from build123d import *

# Parameters (mm, degrees)
BOSS_EXTRUDE1_DEPTH     = 32.5
SKETCH4_R               = 1.05
BOSS_EXTRUDE2_DEPTH     = 2.5
SKETCH5_R               = 1.05
BOSS_EXTRUDE3_DEPTH     = 3
CUT_EXTRUDE1_DEPTH      = 31.122
SKETCH13_W              = 30.122
SKETCH13_H              = 38
BOSS_EXTRUDE7_DEPTH     = 2.5
BOSS_EXTRUDE4_DEPTH     = 5
BOSS_EXTRUDE6_DEPTH     = 5
CUT_EXTRUDE2_DEPTH      = 6
SKETCH14_W              = 15
SKETCH14_H              = 5
CUT_EXTRUDE3_DEPTH      = 11
SKETCH15_W              = 30.122
SKETCH15_H              = 34.5
SKETCH15_R              = 2.495
BOSS_EXTRUDE8_DEPTH     = 3
SKETCH17_R              = 13.75
CUT_EXTRUDE4_DEPTH      = 53
SKETCH19_W              = 15
SKETCH19_H              = 3
CUT_EXTRUDE6_DEPTH      = 30.5
CUT_EXTRUDE6_DEPTH_BACK = 11
SKETCH21_R              = 2.25
CUT_EXTRUDE8_DEPTH      = 1.5
SKETCH20_R              = 10
CUT_EXTRUDE7_DEPTH      = 6
CHAMFER1_SIZE           = 2
CHAMFER1_SIZE2          = 1.154700538
CHAMFER1_PART_2_SIZE    = 2
CHAMFER1_PART_2_SIZE2   = 1.154700538
CHAMFER1_PART_3_SIZE    = 2
CHAMFER1_PART_3_SIZE2   = 1.154700538
CHAMFER1_PART_4_SIZE    = 2
CHAMFER1_PART_4_SIZE2   = 1.154700538
CHAMFER1_PART_5_SIZE    = 2
CHAMFER1_PART_5_SIZE2   = 1.154700538
CHAMFER1_PART_6_SIZE    = 2
CHAMFER1_PART_6_SIZE2   = 1.154700538
CHAMFER1_PART_7_SIZE    = 2
CHAMFER1_PART_7_SIZE2   = 1.154700538
CHAMFER1_PART_8_SIZE    = 2
CHAMFER1_PART_8_SIZE2   = 1.154700538
CHAMFER1_PART_9_SIZE    = 2
CHAMFER1_PART_9_SIZE2   = 1.154700538
CHAMFER1_PART_10_SIZE   = 2
CHAMFER1_PART_10_SIZE2  = 1.154700538
CHAMFER1_PART_11_SIZE   = 2
CHAMFER1_PART_11_SIZE2  = 1.154700538
CHAMFER1_PART_12_SIZE   = 2
CHAMFER1_PART_12_SIZE2  = 1.154700538
CHAMFER1_PART_13_SIZE   = 2
CHAMFER1_PART_13_SIZE2  = 1.154700538
CHAMFER1_PART_14_SIZE   = 2
CHAMFER1_PART_14_SIZE2  = 1.154700538
CHAMFER1_PART_15_SIZE   = 2
CHAMFER1_PART_15_SIZE2  = 1.154700538
CHAMFER1_PART_16_SIZE   = 2
CHAMFER1_PART_16_SIZE2  = 1.154700538
CHAMFER1_PART_17_SIZE   = 2
CHAMFER1_PART_17_SIZE2  = 1.154700538
CHAMFER1_PART_18_SIZE   = 2
CHAMFER1_PART_18_SIZE2  = 1.154700538


with BuildPart() as part:
    # Sketch2 → Boss-Extrude1 (new body)
    with BuildSketch(Plane(origin=(0, 0, 0), x_dir=(1, 0, 0), z_dir=(0, 1, 0))):
        Polygon((15.061, 0), (15.061, 32), (12.561, 32), (12.561, 2.5), (-12.561, 2.5), (-12.561, 32), (-15.061, 32), (-15.061, 0), align=None)
    extrude(amount=BOSS_EXTRUDE1_DEPTH)

    # Sketch4 → Boss-Extrude2 (add)
    with BuildSketch(Plane.XZ):
        Polygon((-7.561, -6), (-7.561, 0), (-15.061, 0), (-15.061, -32), (-12.561, -32), (-12.561, -10), align=None)
        with Locations((-10.2499, -4.95)):
            Circle(SKETCH4_R, mode=Mode.SUBTRACT)
        Polygon((12.561, -10), (7.561, -6), (7.561, 0), (15.061, 0), (15.061, -32), (12.561, -32), align=None)
        with Locations((10.2499, -4.95)):
            Circle(SKETCH4_R, mode=Mode.SUBTRACT)
    extrude(amount=BOSS_EXTRUDE2_DEPTH)

    # Sketch5 → Boss-Extrude3 (add)
    with BuildSketch(Plane(origin=(0, 32.5, 0), x_dir=(1, 0, 0), z_dir=(0, 1, 0))):
        Polygon((-15.061, 32), (-10.2499, 32), (-6.25, 26), (6.25, 26), (10.2499, 32), (15.061, 32), (15.061, 0), (-15.061, 0), align=None)
        with Locations((-10.2499, 8.7)):
            Circle(SKETCH5_R, mode=Mode.SUBTRACT)
        with Locations((10.2499, 8.7)):
            Circle(SKETCH5_R, mode=Mode.SUBTRACT)
    extrude(amount=BOSS_EXTRUDE3_DEPTH)

    # Sketch6 → Cut-Extrude1 (cut, through all)
    with BuildSketch(Plane.ZY.offset(15.061)):
        Polygon((-12.5, 35.5), (-32, 2.5), (-32, 35.5), align=None)
    extrude(amount=-CUT_EXTRUDE1_DEPTH, mode=Mode.SUBTRACT)

    # Sketch13 → Boss-Extrude7 (add)
    with BuildSketch(Plane.XY):
        with Locations((0, 16.5)):
            Rectangle(SKETCH13_W, SKETCH13_H)
    extrude(amount=BOSS_EXTRUDE7_DEPTH)

    # Sketch8 → Boss-Extrude4 (add)
    with BuildSketch(Plane.XY.offset(2.5)):
        Polygon((0, -43.5), (-43.59255168, 16.5), (43.59255168, 16.5), align=None)
    extrude(amount=BOSS_EXTRUDE4_DEPTH)

    # Sketch9 → Boss-Extrude6 (add)
    with BuildSketch(Plane.XY.offset(2.5)):
        Polygon((43.59255168, 16.5), (65.38882752, 46.5), (-65.38882752, 46.5), (-43.59255168, 16.5), align=None)
    extrude(amount=BOSS_EXTRUDE6_DEPTH)

    # Sketch10 → Cut-Extrude2 (cut, through all)
    with BuildSketch(Plane(origin=(0, 0, 2.5), x_dir=(-1, 0, 0), z_dir=(0, 0, -1))):
        Polygon((-25.38882752, 46.5), (-65.38882752, 46.5), (-41.877417429, 14.139320225), align=None)
        Polygon((65.38882752, 46.5), (41.877417429, 14.139320225), (25.38882752, 46.5), align=None)
    extrude(amount=-CUT_EXTRUDE2_DEPTH, mode=Mode.SUBTRACT)

    # Sketch14 → Cut-Extrude3 (cut, through all)
    with BuildSketch(Plane(origin=(0, 0, -2.5), x_dir=(-1, 0, 0), z_dir=(0, 0, -1))):
        Polygon((-7.561, -2.5), (7.561, -2.5), (7.561, 0), (12.561, 0), (12.561, 7.783674653), (-12.561, 7.783674653), (-12.561, 0), (-7.561, 0), align=None)
        with Locations((0, 38)):
            Rectangle(SKETCH14_W, SKETCH14_H)
    extrude(amount=-CUT_EXTRUDE3_DEPTH, mode=Mode.SUBTRACT)

    # Sketch15 → Boss-Extrude8 (add)
    with BuildSketch(Plane.XZ.offset(2.5)):
        with Locations((0, -14.75)):
            Rectangle(SKETCH15_W, SKETCH15_H)
        with Locations((-10.2499, -4.95)):
            Circle(SKETCH15_R, mode=Mode.SUBTRACT)
        with Locations((10.340989886, -4.95)):
            Circle(SKETCH15_R, mode=Mode.SUBTRACT)
    extrude(amount=BOSS_EXTRUDE8_DEPTH)

    # Sketch17 → Cut-Extrude4 (cut, through all)
    with BuildSketch(Plane.XZ.offset(5.5)):
        with Locations((0, -37.5)):
            Circle(SKETCH17_R)
    extrude(amount=-CUT_EXTRUDE4_DEPTH, mode=Mode.SUBTRACT)

    # Sketch19 → Cut-Extrude6 (cut, two sides)
    with BuildSketch(Plane(origin=(0, 0, -2.5), x_dir=(-1, 0, 0), z_dir=(0, 0, -1))) as cut_extrude6_sk:
        with Locations((0, 34)):
            Rectangle(SKETCH19_W, SKETCH19_H)
    extrude(amount=CUT_EXTRUDE6_DEPTH, mode=Mode.SUBTRACT)
    extrude(cut_extrude6_sk.sketch, amount=-CUT_EXTRUDE6_DEPTH_BACK, mode=Mode.SUBTRACT)

    # Sketch21 → Cut-Extrude8 (cut)
    with BuildSketch(Plane(origin=(0, 35.5, 0), x_dir=(1, 0, 0), z_dir=(0, 1, 0))):
        with Locations((-10.2499, 8.7)):
            Circle(SKETCH21_R)
        with Locations((10.2499, 8.7)):
            Circle(SKETCH21_R)
    extrude(amount=-CUT_EXTRUDE8_DEPTH, mode=Mode.SUBTRACT)

    # Sketch20 → Cut-Extrude7 (cut, through all)
    with BuildSketch(Plane(origin=(0, 0, 2.5), x_dir=(-1, 0, 0), z_dir=(0, 0, -1))):
        with Locations((0, -43.5)):
            Circle(SKETCH20_R)
    extrude(amount=-CUT_EXTRUDE7_DEPTH, mode=Mode.SUBTRACT)

    # Chamfer1
    chamfer1_edges = [part.edges().sort_by_distance(p)[0] for p in [
        (-23.877634976, -10.635254916, 7.5),
    ]]
    chamfer1_side = [part.faces().sort_by_distance(p)[0] for p in [
        (-23.877634976, -10.635254916, 5),
    ]]
    chamfer(chamfer1_edges, length=CHAMFER1_SIZE, length2=CHAMFER1_SIZE2, reference=chamfer1_side[0])

    # Chamfer1 part 2
    chamfer1_part_2_edges = [part.edges().sort_by_distance(p)[0] for p in [
        (-33.633122475, 30.319660113, 7.5),
    ]]
    chamfer1_part_2_side = [part.faces().sort_by_distance(p)[0] for p in [
        (-33.633122475, 30.319660113, 5),
    ]]
    chamfer(chamfer1_part_2_edges, length=CHAMFER1_PART_2_SIZE, length2=CHAMFER1_PART_2_SIZE2, reference=chamfer1_part_2_side[0])

    # Chamfer1 part 3
    chamfer1_part_3_edges = [part.edges().sort_by_distance(p)[0] for p in [
        (0, 46.5, 7.5),
    ]]
    chamfer1_part_3_side = [part.faces().sort_by_distance(p)[0] for p in [
        (0, 46.5, 5),
    ]]
    chamfer(chamfer1_part_3_edges, length=CHAMFER1_PART_3_SIZE, length2=CHAMFER1_PART_3_SIZE2, reference=chamfer1_part_3_side[0])

    # Chamfer1 part 4
    chamfer1_part_4_edges = [part.edges().sort_by_distance(p)[0] for p in [
        (33.633122475, 30.319660113, 7.5),
    ]]
    chamfer1_part_4_side = [part.faces().sort_by_distance(p)[0] for p in [
        (33.633122475, 30.319660113, 5),
    ]]
    chamfer(chamfer1_part_4_edges, length=CHAMFER1_PART_4_SIZE, length2=CHAMFER1_PART_4_SIZE2, reference=chamfer1_part_4_side[0])

    # Chamfer1 part 5
    chamfer1_part_5_edges = [part.edges().sort_by_distance(p)[0] for p in [
        (23.877634976, -10.635254916, 7.5),
    ]]
    chamfer1_part_5_side = [part.faces().sort_by_distance(p)[0] for p in [
        (23.877634976, -10.635254916, 5),
    ]]
    chamfer(chamfer1_part_5_edges, length=CHAMFER1_PART_5_SIZE, length2=CHAMFER1_PART_5_SIZE2, reference=chamfer1_part_5_side[0])

    # Chamfer1 part 6
    chamfer1_part_6_edges = [part.edges().sort_by_distance(p)[0] for p in [
        (0, -33.5, 7.5),
    ]]
    chamfer1_part_6_side = [part.faces().sort_by_distance(p)[0] for p in [
        (0, -33.5, 5),
    ]]
    chamfer(chamfer1_part_6_edges, length=CHAMFER1_PART_6_SIZE, length2=CHAMFER1_PART_6_SIZE2, reference=chamfer1_part_6_side[0])

    # Chamfer1 part 7
    chamfer1_part_7_edges = [part.edges().sort_by_distance(p)[0] for p in [
        (7.5, 36.5, 7.5),
    ]]
    chamfer1_part_7_side = [part.faces().sort_by_distance(p)[0] for p in [
        (7.5, 35.125615764, -0.682301365),
    ]]
    chamfer(chamfer1_part_7_edges, length=CHAMFER1_PART_7_SIZE, length2=CHAMFER1_PART_7_SIZE2, reference=chamfer1_part_7_side[0])

    # Chamfer1 part 8
    chamfer1_part_8_edges = [part.edges().sort_by_distance(p)[0] for p in [
        (0, 40.5, 7.5),
    ]]
    chamfer1_part_8_side = [part.faces().sort_by_distance(p)[0] for p in [
        (0, 40.5, 5),
    ]]
    chamfer(chamfer1_part_8_edges, length=CHAMFER1_PART_8_SIZE, length2=CHAMFER1_PART_8_SIZE2, reference=chamfer1_part_8_side[0])

    # Chamfer1 part 9
    chamfer1_part_9_edges = [part.edges().sort_by_distance(p)[0] for p in [
        (-7.5, 36.5, 7.5),
    ]]
    chamfer1_part_9_side = [part.faces().sort_by_distance(p)[0] for p in [
        (-7.5, 35.125615764, -0.682301365),
    ]]
    chamfer(chamfer1_part_9_edges, length=CHAMFER1_PART_9_SIZE, length2=CHAMFER1_PART_9_SIZE2, reference=chamfer1_part_9_side[0])

    # Chamfer1 part 10
    chamfer1_part_10_edges = [part.edges().sort_by_distance(p)[0] for p in [
        (12.561, 3.891837327, 7.5),
    ]]
    chamfer1_part_10_side = [part.faces().sort_by_distance(p)[0] for p in [
        (12.561, 11.913281954, -12.779758376),
    ]]
    chamfer(chamfer1_part_10_edges, length=CHAMFER1_PART_10_SIZE, length2=CHAMFER1_PART_10_SIZE2, reference=chamfer1_part_10_side[0])

    # Chamfer1 part 11
    chamfer1_part_11_edges = [part.edges().sort_by_distance(p)[0] for p in [
        (0, -2.5, 7.5),
    ]]
    chamfer1_part_11_side = [part.faces().sort_by_distance(p)[0] for p in [
        (0, -2.5, -11.382409491),
    ]]
    chamfer(chamfer1_part_11_edges, length=CHAMFER1_PART_11_SIZE, length2=CHAMFER1_PART_11_SIZE2, reference=chamfer1_part_11_side[0])

    # Chamfer1 part 12
    chamfer1_part_12_edges = [part.edges().sort_by_distance(p)[0] for p in [
        (-7.561, -1.25, 7.5),
    ]]
    chamfer1_part_12_side = [part.faces().sort_by_distance(p)[0] for p in [
        (-7.561, -1.25, 0.75),
    ]]
    chamfer(chamfer1_part_12_edges, length=CHAMFER1_PART_12_SIZE, length2=CHAMFER1_PART_12_SIZE2, reference=chamfer1_part_12_side[0])

    # Chamfer1 part 13
    chamfer1_part_13_edges = [part.edges().sort_by_distance(p)[0] for p in [
        (7.561, -1.25, 7.5),
    ]]
    chamfer1_part_13_side = [part.faces().sort_by_distance(p)[0] for p in [
        (7.561, -1.25, 0.75),
    ]]
    chamfer(chamfer1_part_13_edges, length=CHAMFER1_PART_13_SIZE, length2=CHAMFER1_PART_13_SIZE2, reference=chamfer1_part_13_side[0])

    # Chamfer1 part 14
    chamfer1_part_14_edges = [part.edges().sort_by_distance(p)[0] for p in [
        (-10.061, 0, 7.5),
    ]]
    chamfer1_part_14_side = [part.faces().sort_by_distance(p)[0] for p in [
        (-10.164720046, 0, -0.075145261),
    ]]
    chamfer(chamfer1_part_14_edges, length=CHAMFER1_PART_14_SIZE, length2=CHAMFER1_PART_14_SIZE2, reference=chamfer1_part_14_side[0])

    # Chamfer1 part 15
    chamfer1_part_15_edges = [part.edges().sort_by_distance(p)[0] for p in [
        (10.061, 0, 7.5),
    ]]
    chamfer1_part_15_side = [part.faces().sort_by_distance(p)[0] for p in [
        (10.164720046, 0, -0.075145261),
    ]]
    chamfer(chamfer1_part_15_edges, length=CHAMFER1_PART_15_SIZE, length2=CHAMFER1_PART_15_SIZE2, reference=chamfer1_part_15_side[0])

    # Chamfer1 part 16
    chamfer1_part_16_edges = [part.edges().sort_by_distance(p)[0] for p in [
        (-12.561, 3.891837327, 7.5),
    ]]
    chamfer1_part_16_side = [part.faces().sort_by_distance(p)[0] for p in [
        (-12.561, 11.913281954, -12.779758376),
    ]]
    chamfer(chamfer1_part_16_edges, length=CHAMFER1_PART_16_SIZE, length2=CHAMFER1_PART_16_SIZE2, reference=chamfer1_part_16_side[0])

    # Chamfer1 part 17
    chamfer1_part_17_edges = [part.edges().sort_by_distance(p)[0] for p in [
        (0, 7.783674653, 7.5),
    ]]
    chamfer1_part_17_side = [part.faces().sort_by_distance(p)[0] for p in [
        (0, 7.783674653, 2.5),
    ]]
    chamfer(chamfer1_part_17_edges, length=CHAMFER1_PART_17_SIZE, length2=CHAMFER1_PART_17_SIZE2, reference=chamfer1_part_17_side[0])

    # Chamfer1 part 18
    chamfer1_part_18_edges = [part.edges().sort_by_distance(p)[0] for p in [
        (0, 32.5, 7.5),
    ]]
    chamfer1_part_18_side = [part.faces().sort_by_distance(p)[0] for p in [
        (0, 32.5, 2.5),
    ]]
    chamfer(chamfer1_part_18_edges, length=CHAMFER1_PART_18_SIZE, length2=CHAMFER1_PART_18_SIZE2, reference=chamfer1_part_18_side[0])


solid = part.part
Input: part model. Units: mm. Frame: model coordinates. A direction names the side the tool comes from. Give positions to 0.01 mm unless a question says otherwise; leave off trailing zeros. Loops run counter-clockwise (first coordinate to the right, second up) from the corner with the lowest first, then second, coordinate; pieces in that order, holes last. Notation, with made-up numbers: (-29.5, 22.5) - (-16.5, 22.5) arc R26 cw to (-16.5, 41.5) - close; hole circle Ø2 at (75.5, 16). An arc over 180 degrees is marked (long way). Use CSV: the item, a comma, the result in double quotes. Start each with the question number.
Item 1: Mould query, pull axis Z, two halves, no side actions, for faces 1 (the flat face through (-10.1, -1.23, -8.03)), 2 (the cylindrical face through (9.2, -1.2, -4.9)), 3 (the flat face through (-33.75, 30.09, 3.98)). Classes: pulls with the +Z half, pulls with the -Z half, needs draft (parallel to the pull), parting line crosses it, or undercut.
Item 2: Reachability of faces 4 (the cylindrical face through (11.288, 34.76, -6.704)), 5 (the flat face through (7.561, -1, 0)), 6 (the flat face through (11, -2.5, -4)) from +Z, -Z, +X, -X, +Y, -Y: full face, straight path, thin tool, end or side. Return the list, or none.
Item 3: Section A-A on z = 0. Return loops of the section in (x, y).
Item 4: Section C-C on z = -26.5. Return loops of the section in (x, y).
Item 5: Section D-D on x = -17. Return loops of the section in (y, z), then the cut area to 3 significant figures.
Item 6: Line query: line 1 (X direction, y = -0.5, z = -5); line 2 (Y direction, x = 0, z = 4); line 3 (X direction, y = 34.4, z = -8.7). Output: solid intervals per line, ascending.
Item 7: Contact query for flat-ended pins moving along their axis: P1, Ø3.5, axis at x = -10.25, z = -8.7, coming from the -Y side; P2, Ø4, axis at x = -26.5, y = 10, coming from the -Z side; P3, Ø1.2, axis at y = -1, z = 2.5, coming from the +X side; P4, Ø9, axis at x = 2, z = 2, coming from the -Y side. Output: stop coordinate, or through.
Item 8: Section B-B on z = -4.95. State how many separate pieces and enclosed holes the cut face has, then the cut area to 3 significant figures.
Ans:
1,face 1,"pulls with the -Z half"
1,face 2,"undercut"
1,face 3,"needs draft"
2,face 4,"+Y"
2,face 5,"+Z, -Z"
2,face 6,"-Y"
3,outline,"(-15.06, -5.5) - (15.06, -5.5) - (15.06, 35.5) - (7.5, 35.5) - (7.5, 32.5) - (-7.5, 32.5) - (-7.5, 35.5) - (-15.06, 35.5) - close; hole (-12.56, 0) - (-7.56, 0) - (-7.56, -2.5) - (7.56, -2.5) - (7.56, 0) - (12.56, 0) - (12.56, 7.78) - (-12.56, 7.78) - close"
4,outline,"(-15.06, -5.5) - (-8.25, -5.5) - (-8.25, -2.5) - (-12.56, -2.5) - (-12.56, 11.81) - (-15.06, 11.81) - close; (8.25, -5.5) - (15.06, -5.5) - (15.06, 11.81) - (12.56, 11.81) - (12.56, -2.5) - (8.25, -2.5) - close"
5,outline,"(-20.1, 2.5) - (46.5, 2.5) - (46.5, 5.5) - (45.35, 7.5) - (-18.14, 7.5) - (-20.1, 5.5) - close"
5,area,"330 mm2"
6,line 1,"x = -15.06 to -11.3, -9.2 to -7.56, 7.56 to 9.2, 11.3 to 15.06"
6,line 2,"y = -33.5 to -2.5, 7.78 to 32.5, 40.5 to 46.5"
6,line 3,"x = -15.06 to -12.5, -8 to -7.5, 7.5 to 8, 12.5 to 15.06"
7,P1,"stops at y = -5.5"
7,P2,"stops at z = 2.5"
7,P3,"stops at x = 31.31"
7,P4,"stops at y = -35.41"
8,separate pieces,"3"
8,enclosed holes,"0"
8,area,"295 mm2"
